Check sheet for the modelled part. Datum: model origin and axes. Units: mm. A direction names the side the tool comes from. Round coordinates to 2 decimals unless told otherwise and drop trailing zeros. Write each loop counter-clockwise with the first axis right and the second up, starting at its lowest first coordinate (ties: lowest second). Pieces come first, ordered by that corner, then holes. Notation, with made-up numbers: (-40, 14) - (1, 14) arc R14 cw to (1, 18) - close; hole circle Ø10 at (65, 16.25). An arc over 180 degrees is marked (long way). Answer as a JSON object with one key per item and string values. Group by question number.
Item 1: Set-up check for faces 1 (the flat face through (71, 2, -2)), 2 (the flat face through (9, 2, 17)), 3 (the flat face through (5, 2, 0)), 4 (the flat face through (78, 2, 37.75)): record each of +Z, -Z, +X, -X, +Y, -Y from which the full face is reachable in a straight line by a thin tool's end or side.
Item 2: Sectioned sample at B-B on y = 0.95. Count the separate pieces of the cut face and the enclosed holes in it, plus the area to 3 significant figures.
Item 3: Gauge pin test, flat ends, axial feed: P1, Ø1.2, axis at y = 2.5, z = 42.5, coming from the -X side; P2, Ø1, axis at x = 45, y = 0.5, coming from the +Z side; P3, Ø2, axis at y = 2, z = 34, coming from the +X side. Record the tip position at first contact, or that the pin passes through.
Item 4: Release check for a two-part mould opening along X. For faces 5 (the flat face through (78, 2, 2.75)), 6 (the flat face through (66, 2, 40.5)), 7 (the flat face through (81, 2, 13)), 8 (the flat face through (0, 2, 21)) record: pulls with the +X half, pulls with the -X half, needs draft (parallel to the pull), parting line crosses it, or undercut.
Item 5: Thickness scan on line 1 (Z direction, x = 7.5, y = 0.65); line 2 (X direction, y = 2.85, z = 17); line 3 (Z direction, x = 63, y = 1.7). Record the ranges inside material, lowest first.
Item 6: Sectioned sample at A-A on x = 7. Record the boundary of the cut face in (y, z), plus the area to 3 significant figures.
Item 7: Sectioned sample at C-C on x = 70. Record the boundary of the cut face in (y, z), plus the area to 3 significant figures.
```python
from build123d import *

# Parameters (mm, degrees)
SKETCH1_W           = 75
SKETCH1_H           = 40.5
BOSS_EXTRUDE1_DEPTH = 4
SKETCH2_W           = 2.75
SKETCH2_H           = 4
SKETCH2_W_2         = 10
BOSS_EXTRUDE2_DEPTH = 6
SKETCH3_W           = 10
SKETCH3_H           = 4
BOSS_EXTRUDE3_DEPTH = 4
LPATTERN1_COUNT     = 4
LPATTERN1_PITCH     = 20
SKETCH4_W           = 3
SKETCH4_H           = 1.5
CUT_EXTRUDE1_DEPTH  = 5


with BuildPart() as part:
    # Sketch1 → Boss-Extrude1 (new body)
    with BuildSketch(Plane(origin=(0, 0, 0), x_dir=(1, 0, 0), z_dir=(0, 1, 0))):
        with Locations((37.5, -20.25)):
            Rectangle(SKETCH1_W, SKETCH1_H)
    extrude(amount=BOSS_EXTRUDE1_DEPTH)

    # Sketch2 → Boss-Extrude2 (add)
    with BuildSketch(Plane(origin=(75, 0, 0), x_dir=(0, 0, -1), z_dir=(1, 0, 0))):
        with Locations((-39.125, 2)):
            Rectangle(SKETCH2_W, SKETCH2_H)
        with Locations((-27.75, 2)):
            Rectangle(SKETCH2_W_2, SKETCH2_H)
        with Locations((-12.75, 2)):
            Rectangle(SKETCH2_W_2, SKETCH2_H)
        with Locations((-1.375, 2)):
            Rectangle(SKETCH2_W, SKETCH2_H)
    extrude(amount=BOSS_EXTRUDE2_DEPTH)

    # Sketch3 → Boss-Extrude3 (add, through all)
    with BuildSketch(Plane(origin=(0, 4, 0), x_dir=(1, 0, 0), z_dir=(0, 1, 0))):
        with Locations((76, 2)):
            Rectangle(SKETCH3_W, SKETCH3_H)
        with Locations((76, -42.5)):
            Rectangle(SKETCH3_W, SKETCH3_H)
    boss_extrude3 = extrude(amount=-BOSS_EXTRUDE3_DEPTH)

    # LPattern1: Boss-Extrude3 ×4
    with Locations(*[(-i * LPATTERN1_PITCH, 0, 0) for i in range(1, LPATTERN1_COUNT)]):
        add(boss_extrude3)

    # Sketch4 → Cut-Extrude1 (cut, through all)
    with BuildSketch(Plane(origin=(0, 4, 0), x_dir=(1, 0, 0), z_dir=(0, 1, 0))):
        with Locations((7.5, -24)):
            Rectangle(SKETCH4_W, SKETCH4_H)
        with Locations((7.5, -16.5)):
            Rectangle(SKETCH4_W, SKETCH4_H)
    extrude(amount=-CUT_EXTRUDE1_DEPTH, mode=Mode.SUBTRACT)


solid = part.part
```
Completed:
{
 "1": {"face 1": "-Z, +Y, -Y", "face 2": "+Y, -Y", "face 3": "-Z, -X, +Y, -Y", "face 4": "+X, +Y, -Y"},
 "2": {"separate pieces": "1", "enclosed holes": "2", "area": "3,500 mm²"},
 "3": {"P1": "x = 11", "P2": "z = 40.5", "P3": "x = 75"},
 "4": {"face 5": "needs draft", "face 6": "undercut", "face 7": "pulls with the +X half", "face 8": "pulls with the -X half"},
 "5": {"line 1": "0 to 15.75, 17.25 to 23.25, 24.75 to 40.5", "line 2": "0 to 6, 9 to 81", "line 3": "0 to 40.5"},
 "6": {"outline": "(0, 0) - (4, 0) - (4, 15.75) - (0, 15.75) - close; (0, 17.25) - (4, 17.25) - (4, 23.25) - (0, 23.25) - close; (0, 24.75) - (4, 24.75) - (4, 40.5) - (0, 40.5) - close", "area": "150 mm²"},
 "7": {"outline": "(0, 0) - (4, 0) - (4, 40.5) - (0, 40.5) - close", "area": "162 mm²"}
}
